Source: CAD feature listing. Evaluate the final solid. Frame: model axes, mm. Face numbers are marked on the shaded views. Round coordinates to 2 decimals unless told otherwise and drop trailing zeros. Loops run counter-clockwise (first coordinate to the right, second up) from the corner with the lowest first, then second, coordinate; pieces in that order, holes last. Notation, with made-up numbers: (33.25, 13) -> (41.25, 13) arc R21 cw to (41.25, 41) -> close; hole circle Ø9 at (61, 18). An arc over 180 degrees is marked (long way). Return JSON: item names as keys, results as strings. Group by question number.
```python
from build123d import *

# Parameters (mm, degrees)
SKETCH_R     = 40.2
SKETCH_R_2   = 22.5
PAD_DEPTH    = 5
PAD001_DEPTH = 74
POCKET_DEPTH = 5
FILLET_R     = 1.5
FILLET001_R  = 5.4
SKETCH003_R  = 1.8
HOLE_DEPTH   = 5
CHAMFER_SIZE = 0.4


with BuildPart() as part:
    # Sketch → Pad (new body)
    with BuildSketch(Plane.XY):
        Circle(SKETCH_R)
        Circle(SKETCH_R_2, mode=Mode.SUBTRACT)
    extrude(amount=PAD_DEPTH)

    # Sketch001 → Pad001 (join)
    with BuildSketch(Plane.XY):
        with BuildLine():
            ThreePointArc((0, 29.5), (-29.5, 0), (0, -29.5))
            Line((0, -22.5), (0, -29.5))
            ThreePointArc((0, 22.5), (-22.5, 0), (0, -22.5))
            Line((0, 29.5), (0, 22.5))
        make_face()
    extrude(amount=PAD001_DEPTH)

    # Sketch002 → Pocket (cut)
    with BuildSketch(Plane.XY):
        with BuildLine():
            ThreePointArc((0, -30), (30, 0), (0, 30))
            Line((0, 30), (0, 22.5))
            ThreePointArc((0, -22.5), (22.5, 0), (0, 22.5))
            Line((0, -22.5), (0, -30))
        make_face()
    extrude(amount=POCKET_DEPTH, mode=Mode.SUBTRACT)

    # Fillet
    fillet_edges = [part.edges().sort_by_distance(p)[0] for p in [
        (0, -29.5, 39.5),
        (0, 29.5, 39.5),
    ]]
    fillet(fillet_edges, radius=FILLET_R)

    # Fillet001
    fillet001_edges = [part.edges().sort_by_distance(p)[0] for p in [
        (-22.5, 0, 74),
        (0, -22.5, 39.5),
        (0, 22.5, 39.5),
    ]]
    fillet(fillet001_edges, radius=FILLET001_R)

    # Sketch003 → Hole (cut)
    with BuildSketch(Plane.XY):
        with Locations((-36.6, 0)):
            Circle(SKETCH003_R)
        with Locations((18.3, 31.69653)):
            Circle(SKETCH003_R)
        with Locations((18.3, -31.69653)):
            Circle(SKETCH003_R)
    extrude(amount=HOLE_DEPTH, mode=Mode.SUBTRACT)

    # Chamfer
    chamfer_edges = [part.edges().sort_by_distance(p)[0] for p in [
        (-40.2, 0, 5),
        (20.1, -31.69653, 5),
        (20.1, 31.69653, 5),
        (30, 0, 5),
        (-40.2, 0, 0),
        (30, 0, 0),
        (20.1, -31.69653, 0),
        (20.1, 31.69653, 0),
        (-34.8, 0, 0),
        (0, -29.75, 0),
        (0, -28.436216, 0),
        (-1.228437, -23.943428, 0),
        (-22.5, 0, 0),
        (-1.228437, 23.943428, 0),
        (0, 29.75, 0),
        (0, 28.436216, 0),
        (-34.8, 0, 5),
    ]]
    chamfer(chamfer_edges, length=CHAMFER_SIZE)


solid = part.part
```
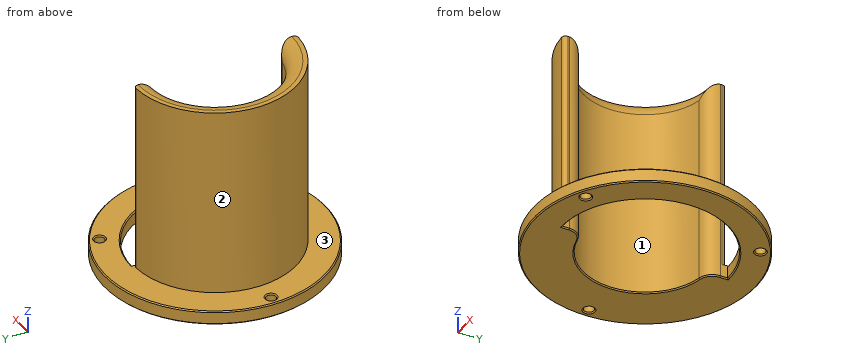
(1) Pin query (flat end, axial travel): pin 1 (1.5 mm diameter, centred on y = 28.5, z = 38, fed in from +X); pin 2 (1 mm diameter, centred on x = -2.5, z = 49.5, fed in from -Y); pin 3 (8 mm diameter, centred on x = -1, z = 22.5, fed in from +Y). Return the tip coordinate at first contact, or that it passes through.
(2) Mould query, pull axis Y, two halves, no side actions, for the marked faces 1, 2 and 3. Classes: released by +Y, released by -Y, zero draft, split by the parting line, or undercut.
(3) Cut plane C-C (x = 18.3). Count the separate pieces of the cut face and the enclosed holes in it, and give its area (3 significant figures).
(4) Cut plane A-A (y = 0). Return loops of the section in (x, z).
(5) Ray query, line 1 (Y direction, x = 18.3, z = 1.4); line 2 (Z direction, x = -1, y = 35); line 3 (Y direction, x = -9.5, z = 4.5). Return the intervals inside material, ascending.
Answers follow:
{
 "1": {"pin 1": "x = 0", "pin 2": "y = -29.43", "pin 3": "y = 29.46"},
 "2": {"face 1": "undercut", "face 2": "split by the parting line", "face 3": "zero draft"},
 "3": {"separate pieces": "4", "enclosed holes": "0", "area": "82.8 mm^2"},
 "4": {"outline": "(-40.2, 0.4) -> (-39.8, 0) -> (-38.8, 0) -> (-38.4, 0.4) -> (-38.4, 4.6) -> (-38.8, 5) -> (-39.8, 5) -> (-40.2, 4.6) -> close; (-34.8, 0.4) -> (-34.4, 0) -> (-22.9, 0) -> (-22.5, 0.4) -> (-22.5, 68.6) arc R5.4 ccw to (-27.9, 74) -> (-29.5, 74) -> (-29.5, 5) -> (-34.4, 5) -> (-34.8, 4.6) -> close; (30, 0.4) -> (30.4, 0) -> (39.8, 0) -> (40.2, 0.4) -> (40.2, 4.6) -> (39.8, 5) -> (30.4, 5) -> (30, 4.6) -> close"},
 "5": {"line 1": "-35.79 to -33.5, -29.9 to -23.77, 23.77 to 29.9, 33.5 to 35.79", "line 2": "0 to 5", "line 3": "-39.06 to -20.4, 20.4 to 39.06"}
}
